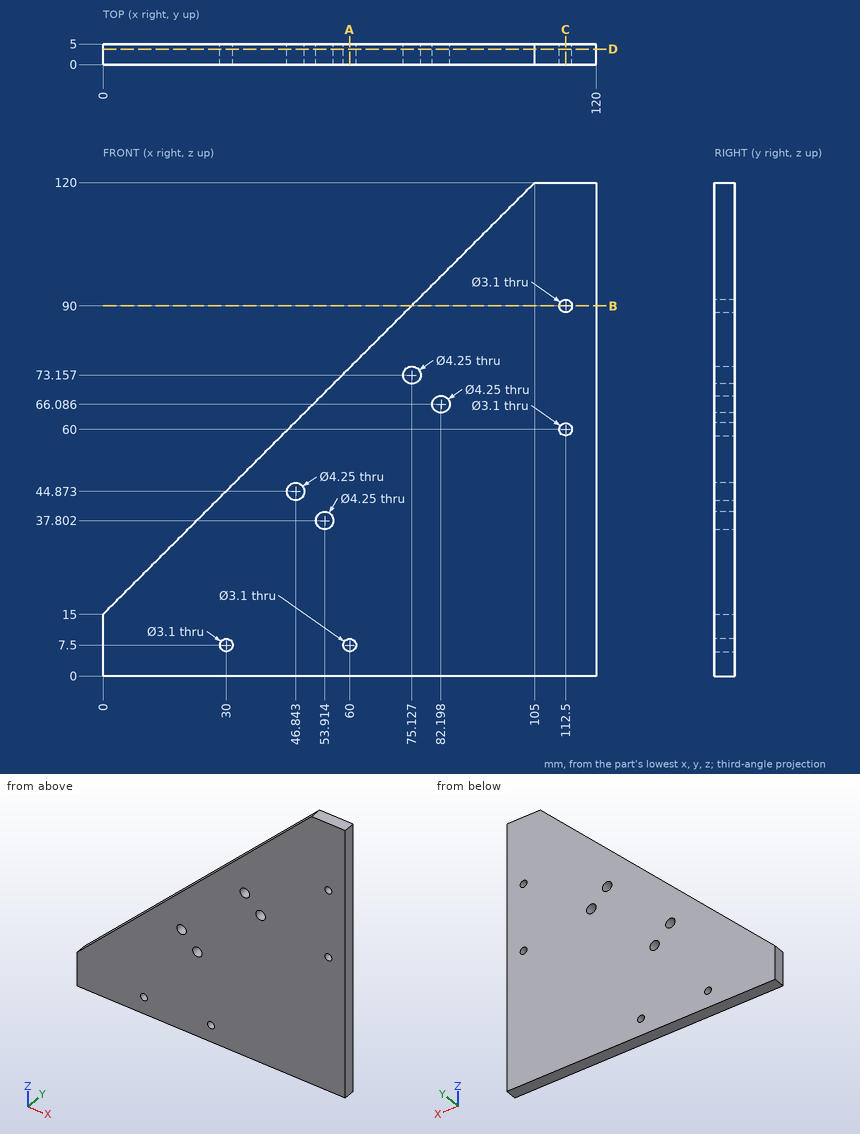
The figure shows three views and two pictorial views of one solid part (mm, origin at its lowest corner). Answer the questions. Coordinates: 2 decimals unless noted, no trailing zeros. Loops run counter-clockwise (first coordinate to the right, second up) from the corner with the lowest first, then second, coordinate; pieces in that order, holes last. Notation, with made-up numbers: (45.5, 6.25) -> (77.5, 6.25) arc R13 cw to (77.5, 20.25) -> close; hole circle Ø7 at (48, 39). An arc over 180 degrees is marked (long way). Return JSON: item names as keys, results as strings. Group by question number.
(1) Find the intervals of material crossed by probe 1 along Z at (x, y) = (111.5, 2.3) (1 decimal); probe 2 along Z at (x, y) = (47, 2.05) (1 decimal); probe 3 along X at (y, z) = (4.2, 38), in increasing order. Write a range as from..to.
(2) A cutting plane is placed at A-A on x = 60. Write down the section's boundary in (y, z).
(3) A cutting plane is placed at D-D on y = 3.75. Count the separate pieces of the cut face and the enclosed holes in it, and give its area (3 significant figures).
(4) A cutting plane is placed at B-B on z = 90. Write down the section's boundary in (x, y).
(5) A cutting plane is placed at C-C on x = 112.5. Write down the section's boundary in (y, z).
The answers:
{
 "1": {"probe 1": "z = 0..58.8, 61.2..88.8, 91.2..120", "probe 2": "z = 0..42.8, 47..62", "probe 3": "x = 23..51.8, 56.03..120"},
 "2": {"outline": "(0, 0) -> (5, 0) -> (5, 5.95) -> (0, 5.95) -> close; (0, 9.05) -> (5, 9.05) -> (5, 75) -> (0, 75) -> close"},
 "3": {"separate pieces": "1", "enclosed holes": "8", "area": "8,800 mm^2"},
 "4": {"outline": "(75, 0) -> (110.95, 0) -> (110.95, 5) -> (75, 5) -> close; (114.05, 0) -> (120, 0) -> (120, 5) -> (114.05, 5) -> close"},
 "5": {"outline": "(0, 0) -> (5, 0) -> (5, 58.45) -> (0, 58.45) -> close; (0, 61.55) -> (5, 61.55) -> (5, 88.45) -> (0, 88.45) -> close; (0, 91.55) -> (5, 91.55) -> (5, 120) -> (0, 120) -> close"}
}
